For this review, take the finished solid that the model builds, in its own axes (mm). Give positions to 0.01 mm unless a question says otherwise; leave off trailing zeros. Loops run counter-clockwise (first coordinate to the right, second up) from the corner with the lowest first, then second, coordinate; pieces in that order, holes last. Notation, with made-up numbers: (7.5, -0.5) - (54.5, -0.5) arc R15 ccw to (54.5, 24.5) - close; hole circle Ø8 at (51.5, -14.5). An arc over 180 degrees is marked (long way). Put each result on its own line as item: value. Start each with the question number.
from build123d import *

# Parameters (mm, degrees)
SKETCH1_W           = 95.25
SKETCH1_H           = 177.8
BOSS_EXTRUDE1_DEPTH = 6.35
SKETCH2_W           = 12.7
SKETCH2_H           = 12.7
CUT_EXTRUDE1_DEPTH  = 7.35
LPATTERN1_COUNT     = 4
LPATTERN1_PITCH     = 25.4
SKETCH3_W           = 12.7
SKETCH3_H           = 6.35
CUT_EXTRUDE2_DEPTH  = 7.35
SKETCH5_W           = 6.35
SKETCH5_H           = 12.7
CUT_EXTRUDE4_DEPTH  = 7.35
LPATTERN2_COUNT     = 4
LPATTERN2_PITCH     = 25.4
SKETCH6_W           = 95.25
SKETCH6_H           = 38.1
CUT_EXTRUDE5_DEPTH  = 7.35
SKETCH7_W           = 12.7
SKETCH7_H           = 6.35
BOSS_EXTRUDE2_DEPTH = 6.35
LPATTERN3_COUNT     = 2
LPATTERN3_PITCH     = 25.4
LPATTERN3_COL_COUNT = 2
LPATTERN3_COL_PITCH = 25.4


with BuildPart() as part:
    # Sketch1 → Boss-Extrude1 (new body)
    with BuildSketch(Plane.XY):
        with Locations((47.625, 88.9)):
            Rectangle(SKETCH1_W, SKETCH1_H)
    extrude(amount=BOSS_EXTRUDE1_DEPTH)

    # Sketch2 → Cut-Extrude1 (cut, through all)
    with BuildSketch(Plane.XY.offset(6.35)):
        with Locations((6.35, 6.35)):
            Rectangle(SKETCH2_W, SKETCH2_H)
        with Locations((88.9, 6.35)):
            Rectangle(SKETCH2_W, SKETCH2_H)
    cut_extrude1 = extrude(amount=-CUT_EXTRUDE1_DEPTH, mode=Mode.SUBTRACT)

    # LPattern1: Cut-Extrude1 ×4
    with Locations(*[(0, i * LPATTERN1_PITCH, 0) for i in range(1, LPATTERN1_COUNT)]):
        add(cut_extrude1, mode=Mode.SUBTRACT)

    # Sketch3 → Cut-Extrude2 (cut, through all)
    with BuildSketch(Plane.XY.offset(6.35)):
        with Locations((34.925, 41.275)):
            Rectangle(SKETCH3_W, SKETCH3_H)
        with Locations((60.325, 41.275)):
            Rectangle(SKETCH3_W, SKETCH3_H)
    extrude(amount=-CUT_EXTRUDE2_DEPTH, mode=Mode.SUBTRACT)

    # Sketch5 → Cut-Extrude4 (cut, through all)
    with BuildSketch(Plane.XY.offset(6.35)):
        with Locations((3.175, 107.95)):
            Rectangle(SKETCH5_W, SKETCH5_H)
        with Locations((92.075, 107.95)):
            Rectangle(SKETCH5_W, SKETCH5_H)
    cut_extrude4 = extrude(amount=-CUT_EXTRUDE4_DEPTH, mode=Mode.SUBTRACT)

    # LPattern2: Cut-Extrude4 ×4
    with Locations(*[(0, i * LPATTERN2_PITCH, 0) for i in range(1, LPATTERN2_COUNT)]):
        add(cut_extrude4, mode=Mode.SUBTRACT)

    # Sketch6 → Cut-Extrude5 (cut, through all)
    with BuildSketch(Plane.XY.offset(6.35)):
        with Locations((47.625, 158.75)):
            Rectangle(SKETCH6_W, SKETCH6_H)
    extrude(amount=-CUT_EXTRUDE5_DEPTH, mode=Mode.SUBTRACT)

    # Sketch7 → Boss-Extrude2 (add)
    with BuildSketch(Plane(origin=(0, 139.7, 0), x_dir=(1, 0, 0), z_dir=(0, 1, 0))):
        with Locations((47.625, -3.175)):
            Rectangle(SKETCH7_W, SKETCH7_H)
    boss_extrude2 = extrude(amount=BOSS_EXTRUDE2_DEPTH)

    # LPattern3: Boss-Extrude2 ×2
    with Locations(*[(i * LPATTERN3_PITCH, 0, 0) for i in range(1, LPATTERN3_COUNT)]):
        add(boss_extrude2)

    # LPattern3 col: Boss-Extrude2 ×2
    with Locations(*[(-i * LPATTERN3_COL_PITCH, 0, 0) for i in range(1, LPATTERN3_COL_COUNT)]):
        add(boss_extrude2)


solid = part.part
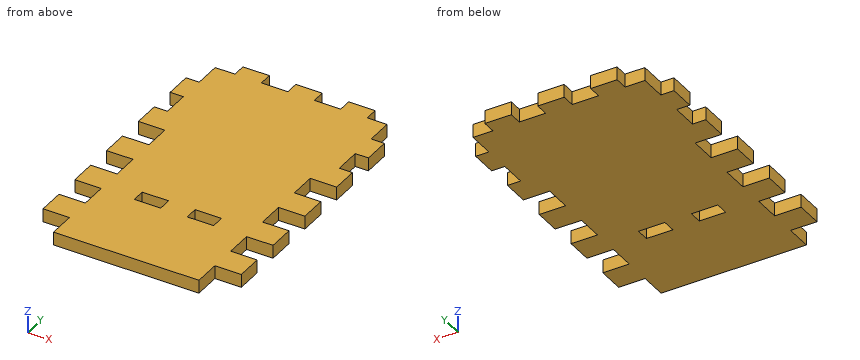
1) Wall thickness on probe 1 along Y at (x, z) = (88.5, 5); probe 2 along X at (y, z) = (41, 2.25) (3 decimals); probe 3 along Y at (x, z) = (65, 2.75): over which ranges is each line inside the solid? List them lowest first.
2) Insertion check: P1, Ø3, axis at y = 33, z = 3.5, coming from the +X side; P2, Ø1.9, axis at x = 34, z = 4, coming from the -Y side; P3, Ø1.9, axis at y = 131.5, z = 1.5, coming from the +X side; P4, Ø1.9, axis at x = 90, z = 2.5, coming from the +Y side. Each pin has a flat end and moves straight along its axis. Give the tip position at first contact, or say it passes through.
3) Take a section at A-A on y = 40.5. State the section outline as (x, z) points (3 decimals), and give its area (3 significant figures).
4) Take a section at C-C on z = 3.25. State how many separate pieces and enclosed holes the cut face has, and give its area (3 significant figures).
5) Take a section at B-B on x = 62. State the section outline as (y, z) points.
6) Take a section at D-D on y = 10. State the section outline as (x, z) points, and give its area (3 significant figures).
Answers follow:
1. probe 1: 12.7 to 25.4, 38.1 to 50.8, 63.5 to 76.2, 88.9 to 139.7
1. probe 2: 0 to 28.575, 41.275 to 53.975, 66.675 to 95.25
1. probe 3: 0 to 38.1, 44.45 to 139.7
2. P1: x = 82.55
2. P2: y = 0
2. P3: x = 88.9
2. P4: y = 127
3. outline: (0, 0) - (28.575, 0) - (28.575, 6.35) - (0, 6.35) - close; (41.275, 0) - (53.975, 0) - (53.975, 6.35) - (41.275, 6.35) - close; (66.675, 0) - (95.25, 0) - (95.25, 6.35) - (66.675, 6.35) - close
3. area: 444 mm2
4. separate pieces: 1
4. enclosed holes: 2
4. area: 11,800 mm2
5. outline: (0, 0) - (38.1, 0) - (38.1, 6.35) - (0, 6.35) - close; (44.45, 0) - (139.7, 0) - (139.7, 6.35) - (44.45, 6.35) - close
6. outline: (12.7, 0) - (82.55, 0) - (82.55, 6.35) - (12.7, 6.35) - close
6. area: 444 mm2
